The model under review builds one solid part; all positions refer to its coordinate system, in mm. A direction names the side the tool comes from. Round coordinates to 2 decimals unless told otherwise and drop trailing zeros. Order: outer loops, then holes, each group sorted by start corner. A loop starts at its lowest first (then second) coordinate and runs counter-clockwise, first axis right, second up. Notation, with made-up numbers: M 35.5,3.5 L 60.5,3.5 A27 cw 60.5,24.5 Z; hole C 43.25,-23.5 d10. An arc over 180 degrees is marked long. Use a Markdown table: item, result. Add a question column.
1. Insertion check: P1, Ø1.5, axis at y = -3.5, z = 17.5, coming from the +X side; P2, Ø4.5, axis at x = 71, z = 9, coming from the -Y side; P3, Ø3, axis at y = 2.5, z = 7.5, coming from the +X side; P4, Ø2, axis at x = 10, y = 2.5, coming from the -Z side. Each pin has a flat end and moves straight along its axis. Give the tip position at first contact, or say it passes through.
2. Consider section B-B on y = -2. State the section outline as (x, z) points.
3. The part is to be moulded in two halves that separate along Z. For faces 4 (the flat face through (-2, -5, 1)), 5 (the cylindrical face through (71.983, -1.056, -6.064)), 6 (the cylindrical face through (-113.648, -3.574, 0.665)), say which applies: +Z half, -Z half, draft (parallel to the pull), parting line (faces both ways), or undercut.
4. For faces 1 (the cylindrical face through (-14.662, -1.958, 1.384)), 2 (the flat face through (0, 3, 20)), 3 (the flat face through (70, 3, -6)), list the 3-axis set-ups (+Z, -Z, +X, -X, +Y, -Y) from which the entire face can be reached by the end or side of a thin tool; tool diameter is ignored.
5. To check wall thickness, follow probe 1 along X at (y, z) = (-0.3, 0); probe 2 along X at (y, z) = (-1.75, -7.5); probe 3 along X at (y, z) = (4, 18). State the ranges of each line that lie inside material, in increasing order.
6. Consider section D-D on z = 0. Count the separate pieces of the cut face and the enclosed holes in it, then the cut area to 3 significant figures.
from build123d import *

# Parameters (mm, degrees)
BOSS_EXTRUDE1_DEPTH     = 5
CUT_EXTRUDE1_DEPTH      = 125.512560278
CUT_EXTRUDE1_DEPTH_BACK = 4
SKETCH2_W               = 46
SKETCH2_H               = 40
SKETCH3_R               = 3
CUT_EXTRUDE2_DEPTH      = 125.25529231
SKETCH4_R               = 2
CUT_EXTRUDE3_DEPTH      = 8
FILLET1_R               = 5


with BuildPart() as part:
    # Sketch1 → Boss-Extrude1 (new, symmetric)
    with BuildSketch(Plane(origin=(0, 0, 0), x_dir=(1, 0, 0), z_dir=(0, 1, 0))):
        with BuildLine():
            Line((-105, -31.676137185), (105, -31.676137185))
            ThreePointArc((105, -31.676137185), (117.249623327, -25.333315035), (119.139622366, -11.669034296))
            Line((119.139622366, -11.669034296), (110.875178831, 11.669034296))
            ThreePointArc((110.875178831, 11.669034296), (101.737771304, 23.739901694), (87.309141554, 28.323862815))
            Line((87.309141554, 28.323862815), (-87.309141554, 28.323862815))
            ThreePointArc((-87.309141554, 28.323862815), (-101.737771304, 23.739901694), (-110.875178831, 11.669034296))
            Line((-110.875178831, 11.669034296), (-119.139622366, -11.669034296))
            ThreePointArc((-119.139622366, -11.669034296), (-117.249623327, -25.333315035), (-105, -31.676137185))
        make_face()
    extrude(amount=BOSS_EXTRUDE1_DEPTH, both=True)

    # Sketch2 → Cut-Extrude1 (cut, two sides: drawn at the far end of the back side and taken through both)
    with BuildSketch(Plane(origin=(0, 5, 0), x_dir=(1, 0, 0), z_dir=(0, 1, 0)).offset(-CUT_EXTRUDE1_DEPTH_BACK)):
        Rectangle(SKETCH2_W, SKETCH2_H)
    extrude(amount=CUT_EXTRUDE1_DEPTH + CUT_EXTRUDE1_DEPTH_BACK, mode=Mode.SUBTRACT)

    # Sketch3 → Cut-Extrude2 (cut, through all)
    with BuildSketch(Plane(origin=(0, 1, 0), x_dir=(1, 0, 0), z_dir=(0, 1, 0))):
        with Locations(Location((12, 0, 0), (0, 0, 270))):
            Circle(SKETCH3_R)
        with Locations(Location((-12, 0, 0), (0, 0, 270))):
            Circle(SKETCH3_R)
    extrude(amount=-CUT_EXTRUDE2_DEPTH, mode=Mode.SUBTRACT)

    # Sketch4 → Cut-Extrude3 (cut)
    with BuildSketch(Plane.XZ.offset(5)):
        with Locations(Location((-70, 9.676137185, 0), (0, 0, 270))):
            Circle(SKETCH4_R)
        with Locations(Location((-70, -6.323862815, 0), (0, 0, 270))):
            Circle(SKETCH4_R)
        with Locations(Location((70, -6.323862815, 0), (0, 0, 270))):
            Circle(SKETCH4_R)
        with Locations(Location((70, 9.676137185, 0), (0, 0, 270))):
            Circle(SKETCH4_R)
    extrude(amount=-CUT_EXTRUDE3_DEPTH, mode=Mode.SUBTRACT)

    # Fillet1
    fillet1_edges = [part.edges().sort_by_distance(p)[0] for p in [
        (101.737771304, -5, -23.739901694),
        (115.007400599, -5, 0),
        (117.249623327, -5, 25.333315035),
        (0, -5, 31.676137185),
        (-117.249623327, -5, 25.333315035),
        (-115.007400599, -5, 0),
        (-101.737771304, -5, -23.739901694),
        (-117.249623327, 5, 25.333315035),
        (-115.007400599, 5, 0),
        (-101.737771304, 5, -23.739901694),
        (0, 5, -28.323862815),
        (101.737771304, 5, -23.739901694),
        (115.007400599, 5, 0),
        (117.249623327, 5, 25.333315035),
        (0, -5, -28.323862815),
        (0, 5, 31.676137185),
    ]]
    fillet(fillet1_edges, radius=FILLET1_R - 0.0001)  # a hair under: the kernel refuses the full size


solid = part.part
Answer block:
| question | item | result |
|---|---|---|
| 1 | P1 | x = 119.15 |
| 1 | P2 | y = -5 |
| 1 | P3 | x = 117.82 |
| 1 | P4 | z = -28.09 |
| 2 | outline | M -118.75,11.81 L -110.48,-11.53 A24.58 ccw -87.31,-27.91 L 87.31,-27.91 A24.58 ccw 110.48,-11.53 L 118.75,11.81 A14.58 ccw 105,31.26 L -105,31.26 A14.58 ccw Z; hole C -70,-6.32 d4; hole C -70,9.68 d4; hole C -12,0 d6; hole C 12,0 d6; hole C 70,-6.32 d4; hole C 70,9.68 d4 |
| 3 | face 4 | draft |
| 3 | face 5 | undercut |
| 3 | face 6 | -Z half |
| 4 | face 1 | +Y, -Y |
| 4 | face 2 | +Y |
| 4 | face 3 | -Y |
| 5 | probe 1 | -115 to -15, -9 to 9, 15 to 115 |
| 5 | probe 2 | -112.02 to -71.62, -68.38 to 68.38, 71.62 to 112.02 |
| 5 | probe 3 | -117.93 to -23, 23 to 117.93 |
| 6 | separate pieces | 3 |
| 6 | enclosed holes | 0 |
| 6 | area | 2,020 mm^2 |
